Can you work these out from the model? Positions are in its coordinate system, mm. A direction names the side the tool comes from. Round coordinates to 2 decimals unless told otherwise and drop trailing zeros. Write each loop counter-clockwise with the first axis right and the second up, starting at its lowest first coordinate (ties: lowest second). Pieces come first, ordered by that corner, then holes.
Q1. For faces 5 (the cylindrical face through (10.6, -77.03, 3.34)), 6 (the flat face through (1, 0, -4)), which set-ups out of +Z, -Z, +X, -X, +Y, -Y let a thin tool reach every point of the face, with its end or its side?
Q2. We'd pull the mould along X, two halves only. Please class faces 1 (the flat face through (0, 19.05, 0)), 2 (the flat face through (0, -66.04, 0)), 3 (the cylindrical face through (-1.487, -87.932, -6.695)), 4 (the cylindrical face through (-0.83, 9.39, 3.72)): +X half, -X half, draft (parallel to the pull), parting line (faces both ways), or undercut.
Q3. I'm going to push flat-ended pins straight in: pin 1 Ø3 at (x, y) = (5.5, -60) entering from -Z; pin 2 Ø5 at (x, z) = (0, -2) entering from -Y; pin 3 Ø6 at (x, y) = (1.5, 4.5) entering from +Z. Where does each tip first touch, or does it pass through?
Q4. If we section it at C-C (y = -86.5): Please give me the cut outline in (x, z) (1 decimal).
Q5. Please list where these lines run through material, in increasing order: line 1 along Z through (x, y) = (0, -95.5); line 2 along Z through (x, y) = (-0.5, -68.5); line 3 along Y through (x, z) = (-7.5, 1.25).
Q6. If we section it at D-D (y = 8): Please give me the cut outline in (x, z), plus the area to 3 significant figures.
from build123d import *

# Parameters (mm, degrees)
F0_R      = 5.715
F1_DEPTH  = 45.72
F3_R      = 11.1125
F4_DEPTH  = 63.5
F6_R      = 6.858
F7_DEPTH  = 43.18
F9_R      = 3.81
F10_DEPTH = 19.05


with BuildPart() as f1:
    # F0 (on Front) → F1 (new body)
    with BuildSketch(Plane.XZ):
        Circle(F0_R)
    extrude(amount=F1_DEPTH)

    # F3 (on offset) → F4 (join)
    with BuildSketch(Plane.XZ.offset(45.72)):
        Circle(F3_R)
    extrude(amount=F4_DEPTH)

    # F6 (on offset) → F7 (cut)
    with BuildSketch(Plane.XZ.offset(109.22)):
        Circle(F6_R)
    extrude(amount=-F7_DEPTH, mode=Mode.SUBTRACT)

    # F9 (on offset) → F10 (join)
    with BuildSketch(Plane(origin=(0, 0, 0), x_dir=(1, 0, 0), z_dir=(0, 1, 0))):
        Circle(F9_R)
    extrude(amount=F10_DEPTH)


solid = f1.part
A:
1. face 5: +Y, -Y
1. face 6: +Y
2. face 1: draft
2. face 2: undercut
2. face 3: undercut
2. face 4: parting line
3. pin 1: stops at z = -10.37
3. pin 2: stops at y = -66.04
3. pin 3: stops at z = 3.81
4. outline: circle Ø22.2 at (0, 0); hole circle Ø13.7 at (0, 0)
5. line 1: z = -11.11 to -6.86, 6.86 to 11.11
5. line 2: z = -11.1 to -6.84, 6.84 to 11.1
5. line 3: y = -109.22 to -45.72
6. outline: circle Ø7.62 at (0, 0)
6. area: 45.6 mm2
